The model under review builds one solid part; all positions refer to its coordinate system, in mm. Face numbers are marked on the shaded views. Coordinates: 2 decimals unless noted, no trailing zeros. Write each loop counter-clockwise with the first axis right and the second up, starting at its lowest first coordinate (ties: lowest second). Pieces come first, ordered by that corner, then holes. Notation, with made-up numbers: (78.5, 21.5) - (92.5, 21.5) arc R14 ccw to (92.5, 46.5) - close; hole circle Ø7 at (31.5, -1). An arc over 180 degrees is marked (long way). Answer as CSV lines item,"result". Start each with the question number.
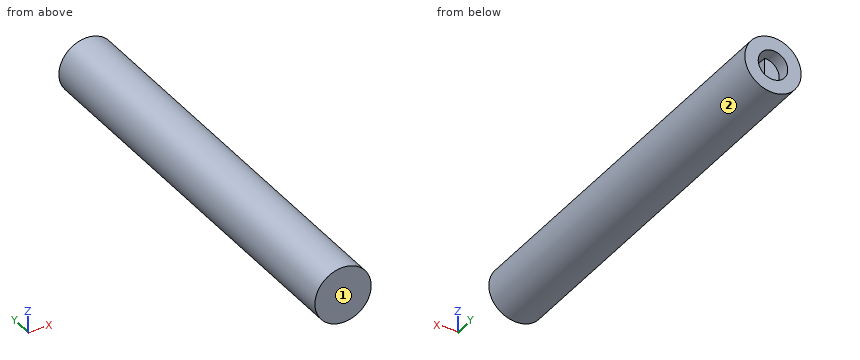
Autodesk Inventor part; units mm, degrees
ref_plane "YZ Plane" through (0, 0, 0) normal (1, 0, 0) x (0, 1, 0)
ref_plane "XZ Plane" through (0, 0, 0) normal (0, 1, 0) x (-1, 0, 0)
ref_plane "XY Plane" through (0, 0, 0) normal (0, 0, 1) x (1, 0, 0)
sketch "スケッチ1" plane through (0, 0, 0) normal (0, 1, 0) x (-1, 0, 0)
  circle A0 centre (0, 0) radius 100
  dimension "d0" = 200
extrude "押し出し1" add sketch "スケッチ1" along normal blind 1500
sketch "スケッチ2" plane through (0, 1500, 0) normal (0, 1, 0) x (1, 0, 0)
  circle A0 centre (0, 0) radius 25
  dimension "d3" = 50
extrude "押し出し2" cut sketch "スケッチ2" against normal blind 50
sketch "スケッチ3" plane through (0, 1500, 0) normal (0, 1, 0) x (1, 0, 0)
  point P0 (0, 0)
sketch "スケッチ4" plane through (0, 1500, 0) normal (0, 1, 0) x (1, 0, 0)
  circle A0 centre (0, 0) radius 25
  circle A1 centre (0, 0) radius 50
  dimension "d6" = 100
extrude "押し出し3" cut sketch "スケッチ4" against normal blind 120 contours A0 | A1
sketch "スケッチ5" plane through (0, 1500, 0) normal (0, 1, 0) x (1, 0, 0)
  circle A0 centre (0, 0) radius 52.5
  dimension "d9" = 105
extrude "押し出し4" cut sketch "スケッチ5" against normal blind 120
sketch "スケッチ6" plane through (0, 1380, 0) normal (0, 1, 0) x (1, 0, 0)
  circle A0 centre (0, 0) radius 52.5
  arc A1 (0.3926, 52.4985) -> (-0.3135, -52.4991) centre (0, 0) ccw
  line L0 (-0.3135, -52.4991) -> (0.3926, 52.4985)
extrude "押し出し5" add sketch "スケッチ6" along normal blind 70 contours L0 A0 picked at (-3.2934, -17.1824)
properties part number "poal1"
(1) The part is to be moulded in two halves that separate along Z. For the marked faces 1 and 2, say which applies: released by +Z, released by -Z, zero draft, split by the parting line, or undercut.
(2) Add section A-A on z = 0. Give the boundary of the cut face in (x, y), then the cut area to 3 significant figures.
(3) Wall thickness on line 1 (Z direction, x = 4.5, y = 1436.5); line 2 (Y direction, x = 19.5, z = 48); line 3 (Y direction, x = -24, z = -27.5): over which ranges is each line inside the solid? List them lowest first.
(4) Add section C-C on z = 82. Give the boundary of the cut face in (x, y).
(5) For pin 1 (4 mm diameter, centred on x = 32, y = 944.5, fed in from +Z); pin 2 (8 mm diameter, centred on y = 747.5, z = -48.5, fed in from +X); pin 3 (3 mm diameter, centred on y = 600, z = -70, fed in from -X), all flat-tipped, find the tip position at first contact; note any pin that passes through.
(6) Add section B-B on y = 1293.5. Give the boundary of the cut face in (x, z).
Reported:
1,face 1,"zero draft"
1,face 2,"split by the parting line"
2,outline,"(-100, 0) - (100, 0) - (100, 1500) - (52.5, 1500) - (52.5, 1380) - (0.04, 1380) - (0.04, 1450) - (-52.5, 1450) - (-52.5, 1500) - (-100, 1500) - close"
2,area,"291,000 mm²"
3,line 1,"-99.9 to -52.31, 52.31 to 99.9"
3,line 2,"0 to 1380"
3,line 3,"0 to 1450"
4,outline,"(-57.24, 0) - (57.24, 0) - (57.24, 1500) - (-57.24, 1500) - close"
5,pin 1,"z = 95.39"
5,pin 2,"x = 89.55"
5,pin 3,"x = -72.85"
6,outline,"circle Ø200 at (0, 0)"
